Model file for the job. Use its own axes, mm. A direction names the side the tool comes from. Give positions to 0.01 mm unless a question says otherwise; leave off trailing zeros. Return JSON: item names as keys, results as strings. Group by question number.
1. Two-plate mould, pull along Z, no slides. Class faces 3 (the face through (49.3, 5.77, -4.71)), 4 (the face through (49, 4.5, 2)), 5 (the face through (49, -10, -7)): released by +Z, released by -Z, zero draft, split by the parting line, or undercut.
2. Wall check: probe 1 along Y at (x, z) = (61, 3.25); probe 2 along Y at (x, z) = (49, 7.25). Give the ranges that are in metal, low to high. Write a range as [from, to].
3. 3-axis set-ups, long thin cutter, end or side, ignore diameter. For faces 1 (the face through (49, -10, 7)), 2 (the face through (49.3, -5.77, 4.71)): which of +Z, -Z, +X, -X, +Y, -Y reach the whole face in a straight line?
4. Pin check, flat tips, straight feed: pin 1 (0.6 mm diameter, centred on x = 30, y = -3, fed in from -Z); pin 2 (8 mm diameter, centred on x = 67.5, z = 1, fed in from -Y); pin 3 (1.6 mm diameter, centred on x = 53, z = 1, fed in from +Y); pin 4 (0.6 mm diameter, centred on x = 69, z = -3, fed in from -Y). Stop position of each tip, or through.
Autodesk Inventor part; units mm, degrees
ref_plane "YZ Plane" through (0, 0, 0) normal (1, 0, 0) x (0, 1, 0)
ref_plane "XZ Plane" through (0, 0, 0) normal (0, 1, 0) x (-1, 0, 0)
ref_plane "XY Plane" through (0, 0, 0) normal (0, 0, 1) x (1, 0, 0)
sketch "Sketch1" plane through (0, 0, 0) normal (1, 0, 0) x (0, 1, 0)
  line L0 (-10, -10) -> (10, 10) construction
  line L1 (10, 10) -> (10, 3.5)
  line L2 (10, 3.5) -> (9.5, 3.5)
  line L3 (9.5, 3.5) -> (9.5, 3)
  line L4 (9.5, 3) -> (8.5, 3)
  line L5 (8.5, 3) -> (8.5, 5.95)
  line L6 (8.5, 5.95) -> (7.0107, 5.95)
  line L7 (7.0107, 5.95) -> (4.5, 3.4393)
  line L8 (4.5, 3.4393) -> (4.5, 0.1525)
  line L9 (2.4501, 2.4501) -> (3.0123, 1.888)
  line L10 (3.0123, 1.888) -> (2.4163, 1.292)
  arc A0 (2.74, 0) -> (2.4163, 1.292) centre (0, 0) ccw
  arc A1 (4.5, 0.1525) -> (4.3475, 0) centre (4.5, 0) ccw
  line L11 (10, 10) -> (2.4501, 2.4501)
  line L12 (4.3475, 0) -> (2.74, 0)
  line L13 (0, 0) -> (2.74, 0) construction
  line L14 (10, 10) -> (3.5, 10)
  line L15 (3.5, 10) -> (3.5, 9.5)
  line L16 (3.5, 9.5) -> (3, 9.5)
  line L17 (3, 9.5) -> (3, 8.5)
  line L18 (3, 8.5) -> (5.95, 8.5)
  line L19 (5.95, 8.5) -> (5.95, 7.0107)
  line L20 (5.95, 7.0107) -> (3.4393, 4.5)
  line L21 (3.4393, 4.5) -> (0.1525, 4.5)
  line L22 (2.4501, 2.4501) -> (1.888, 3.0123)
  line L23 (1.888, 3.0123) -> (1.292, 2.4163)
  arc A2 (1.292, 2.4163) -> (0, 2.74) centre (0, 0) ccw
  arc A3 (0, 4.3475) -> (0.1525, 4.5) centre (0, 4.5) ccw
  line L24 (0, 4.3475) -> (0, 2.74)
  line L25 (0, 0) -> (0, 2.74) construction
  line L26 (-8.5, 5.95) -> (-7.0107, 5.95)
  line L27 (-10, 3.5) -> (-9.5, 3.5)
  line L28 (-8.5, 3) -> (-8.5, 5.95)
  line L29 (-9.5, 3.5) -> (-9.5, 3)
  line L30 (-9.5, 3) -> (-8.5, 3)
  line L31 (-5.95, 8.5) -> (-5.95, 7.0107)
  line L32 (-7.0107, 5.95) -> (-4.5, 3.4393)
  line L33 (-5.95, 7.0107) -> (-3.4393, 4.5)
  line L34 (-10, 10) -> (-10, 3.5)
  line L35 (-10, 10) -> (-3.5, 10)
  line L36 (-10, 10) -> (-2.4501, 2.4501)
  line L37 (-3, 8.5) -> (-5.95, 8.5)
  line L38 (-3, 9.5) -> (-3, 8.5)
  line L39 (-3.5, 10) -> (-3.5, 9.5)
  line L40 (-3.5, 9.5) -> (-3, 9.5)
  line L41 (-3.4393, 4.5) -> (-0.1525, 4.5)
  line L42 (-2.4501, 2.4501) -> (-1.888, 3.0123)
  line L43 (-1.888, 3.0123) -> (-1.292, 2.4163)
  arc A4 (0, 2.74) -> (-1.292, 2.4163) centre (0, 0) ccw
  arc A5 (-0.1525, 4.5) -> (0, 4.3475) centre (0, 4.5) ccw
  line L44 (-2.4501, 2.4501) -> (-3.0123, 1.888)
  line L45 (-4.5, 3.4393) -> (-4.5, 0.1525)
  arc A6 (-4.3475, 0) -> (-4.5, 0.1525) centre (-4.5, 0) ccw
  line L46 (0, 4.3475) -> (0, 2.74)
  line L47 (-4.3475, 0) -> (-2.74, 0)
  arc A7 (-2.4163, 1.292) -> (-2.74, 0) centre (0, 0) ccw
  line L48 (0, 0) -> (0, 2.74) construction
  line L49 (-3.0123, 1.888) -> (-2.4163, 1.292)
  line L50 (-5.95, -8.5) -> (-5.95, -7.0107)
  line L51 (-3.5, -10) -> (-3.5, -9.5)
  line L52 (-3, -8.5) -> (-5.95, -8.5)
  line L53 (-3.5, -9.5) -> (-3, -9.5)
  line L54 (-3, -9.5) -> (-3, -8.5)
  line L55 (-8.5, -5.95) -> (-7.0107, -5.95)
  line L56 (-5.95, -7.0107) -> (-3.4393, -4.5)
  line L57 (-7.0107, -5.95) -> (-4.5, -3.4393)
  line L58 (-10, -10) -> (-3.5, -10)
  line L59 (-10, -10) -> (-10, -3.5)
  line L60 (-10, -10) -> (-2.4501, -2.4501)
  line L61 (-8.5, -3) -> (-8.5, -5.95)
  line L62 (-9.5, -3) -> (-8.5, -3)
  line L63 (-10, -3.5) -> (-9.5, -3.5)
  line L64 (-9.5, -3.5) -> (-9.5, -3)
  line L65 (-4.5, -3.4393) -> (-4.5, -0.1525)
  line L66 (-2.4501, -2.4501) -> (-3.0123, -1.888)
  line L67 (-3.0123, -1.888) -> (-2.4163, -1.292)
  arc A8 (-2.74, 0) -> (-2.4163, -1.292) centre (0, 0) ccw
  arc A9 (-4.5, -0.1525) -> (-4.3475, 0) centre (-4.5, 0) ccw
  line L68 (-2.4501, -2.4501) -> (-1.888, -3.0123)
  line L69 (-3.4393, -4.5) -> (-0.1525, -4.5)
  arc A10 (0, -4.3475) -> (-0.1525, -4.5) centre (0, -4.5) ccw
  line L70 (-4.3475, 0) -> (-2.74, 0)
  line L71 (0, -4.3475) -> (0, -2.74)
  arc A11 (-1.292, -2.4163) -> (0, -2.74) centre (0, 0) ccw
  line L72 (0, 0) -> (-2.74, 0) construction
  line L73 (-1.888, -3.0123) -> (-1.292, -2.4163)
  line L74 (8.5, -5.95) -> (7.0107, -5.95)
  line L75 (10, -3.5) -> (9.5, -3.5)
  line L76 (8.5, -3) -> (8.5, -5.95)
  line L77 (9.5, -3.5) -> (9.5, -3)
  line L78 (9.5, -3) -> (8.5, -3)
  line L79 (5.95, -8.5) -> (5.95, -7.0107)
  line L80 (7.0107, -5.95) -> (4.5, -3.4393)
  line L81 (5.95, -7.0107) -> (3.4393, -4.5)
  line L82 (10, -10) -> (10, -3.5)
  line L83 (10, -10) -> (3.5, -10)
  line L84 (10, -10) -> (2.4501, -2.4501)
  line L85 (3, -8.5) -> (5.95, -8.5)
  line L86 (3, -9.5) -> (3, -8.5)
  line L87 (3.5, -10) -> (3.5, -9.5)
  line L88 (3.5, -9.5) -> (3, -9.5)
  line L89 (3.4393, -4.5) -> (0.1525, -4.5)
  line L90 (2.4501, -2.4501) -> (1.888, -3.0123)
  line L91 (1.888, -3.0123) -> (1.292, -2.4163)
  arc A12 (0, -2.74) -> (1.292, -2.4163) centre (0, 0) ccw
  arc A13 (0.1525, -4.5) -> (0, -4.3475) centre (0, -4.5) ccw
  line L92 (2.4501, -2.4501) -> (3.0123, -1.888)
  line L93 (4.5, -3.4393) -> (4.5, -0.1525)
  arc A14 (4.3475, 0) -> (4.5, -0.1525) centre (4.5, 0) ccw
  line L94 (0, -4.3475) -> (0, -2.74)
  line L95 (4.3475, 0) -> (2.74, 0)
  arc A15 (2.4163, -1.292) -> (2.74, 0) centre (0, 0) ccw
  line L96 (0, 0) -> (0, -2.74) construction
  line L97 (3.0123, -1.888) -> (2.4163, -1.292)
  point P0 (9, 3)
  point P1 (3, 9)
  point P2 (-9, 3)
  point P3 (-3, 9)
  point P4 (-3, -9)
  point P5 (-9, -3)
  point P6 (9, -3)
  point P7 (3, -9)
  dimension "d2" = 6.5
  dimension "d3" = 0.5
  dimension "d4" = 4
  dimension "d5" = 3.465
  dimension "d6" = 5.48
  dimension "d7" = 0.795
  dimension "d8" = 0.305
  dimension "d9" = 2.95
  dimension "d11" = 0.75
  dimension "d14" = 45
  dimension "d15" = 10
  dimension "d16" = 1
  dimension "d17" = 3
  dimension "d18" = 45
  dimension "d21" = 360
extrude "Extrusion1" add sketch "Sketch1" along normal blind 100 contours L1 L2 L3 L4 L5 L6 L7 L8 A1 L12 A0 L10 L9 L11 | L11 L22 L23 A2 L24 A3 L21 L20 L19 L18 L17 L16 L15 L14 | L12 A14 L93 L80 L74 L76 L78 L77 L75 L82 L84 L92 L97 A15 | A4 L43 L42 L36 L35 L39 L40 L38 L37 L31 L33 L41 A5 L24 | L84 L83 L87 L88 L86 L85 L79 L81 L89 A13 L71 A12 L91 L90 | L44 L49 A7 L47 A6 L45 L32 L26 L28 L30 L29 L27 L34 L36 | L71 A10 L69 L56 L50 L52 L54 L53 L51 L58 L60 L68 L73 A11 | A8 L67 L66 L60 L59 L63 L64 L62 L61 L55 L57 L65 A9 L47
properties part number "20mm Extrusion 500mm" material "Aluminum 6061"
Result:
{
 "1": {"face 3": "undercut", "face 4": "undercut", "face 5": "zero draft"},
 "2": {"probe 1": "y = [-9.5, -8.5], [-4.5, 4.5], [8.5, 9.5]", "probe 2": "y = [-10, -5.95], [5.95, 10]"},
 "3": {"face 1": "+Z, -Z, +X, -X, -Y", "face 2": "+X, -X"},
 "4": {"pin 1": "stops at z = -9.5", "pin 2": "stops at y = -10", "pin 3": "stops at y = 4.5", "pin 4": "stops at y = -9.5"}
}
